Part model, mm, in its own coordinate system. Face numbers are marked on the shaded views. A direction names the side the tool comes from. Round coordinates to 2 decimals unless told otherwise and drop trailing zeros. Write each loop counter-clockwise with the first axis right and the second up, starting at its lowest first coordinate (ties: lowest second). Pieces come first, ordered by that corner, then holes.
```python
from build123d import *

# Parameters (mm, degrees)
FILLET2_R = 50.8
FILLET3_R = 7.62


with BuildPart() as part:
    # Sketch1 → Revolve1 (revolve)
    with BuildSketch(Plane(origin=(0, 0, 0), x_dir=(1, 0, 0), z_dir=(0, 1, 0)), mode=Mode.PRIVATE) as revolve1_sk:
        Polygon((-78.74, 0), (-61.722, 0), (-61.722, 147.1422), (0, 147.1422), (0, 294.2844), (-62.23, 294.2844), (-62.23, 249.0724), (-129.54, 249.0724), (-129.54, 37.846), (-78.74, 37.846), align=None)
    revolve(revolve1_sk.sketch.rotate(Axis((0, 0, 0), (0, 0, -1)), 180), axis=Axis((0, 0, 0), (0, 0, -1)))

    # Fillet2
    fillet2_edges = [part.edges().sort_by_distance(p)[0] for p in [
        (-129.54, 0, -37.846),
        (-129.54, 0, -249.0724),
    ]]
    fillet(fillet2_edges, radius=FILLET2_R - 0.0001)  # a hair under: the kernel refuses the full size

    # Fillet3
    fillet3_edges = [part.edges().sort_by_distance(p)[0] for p in [
        (-62.23, 0, -294.2844),
    ]]
    fillet(fillet3_edges, radius=FILLET3_R)


solid = part.part
```
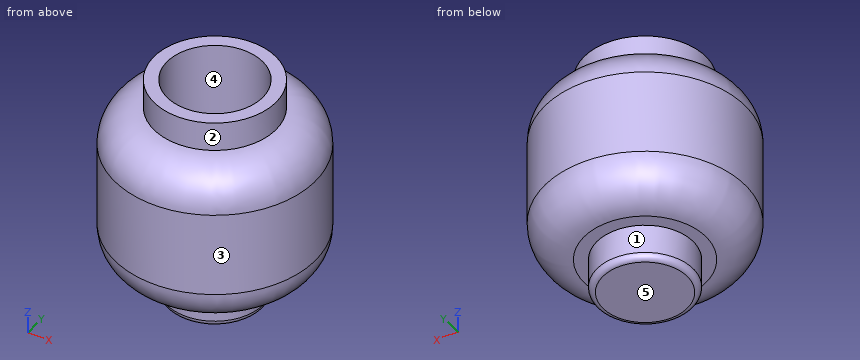
Q1. Cut at D-D on z = -269.5. Write the cut outline in (x, y).
Values follow:
outline: circle Ø124.46 at (0, 0)
Q2. Mould opens along X. For the marked faces 3, 4 and 5 say: +X half, -X half, draft (parallel to the pull), parting line (faces both ways), or undercut.
Values follow:
face 3: parting line
face 4: undercut
face 5: draft
Q3. Wall check: L1, parallel to Y at x = -50, z = -26; L2, parallel to Y at x = 42, z = -78; L3, parallel to Z at x = 3, y = 2.5. Give the ranges that are in metal, low to high.
Values follow:
L1: y = -60.83 to -36.19, 36.19 to 60.83
L2: y = -121.35 to -45.23, 45.23 to 121.35
L3: z = -294.28 to -147.14
Q4. Which spindle directions (+Z, -Z, +X, -X, +Y, -Y) get a long thin tool onto all of the face, cutting with end or side? Do the marked faces 1 and 2. Say none if no direction does.
Values follow:
face 1: -Z
face 2: +Z
Q5. Cut at C-C on z = -177.5. Write the cut outline in (x, y), plus the area to 3 significant figures.
Values follow:
outline: circle Ø259.08 at (0, 0)
area: 52,700 mm2
Q6. Drop flat-ended pins along their axis: pin 1 (8 mm diameter, centred on x = -27.5, z = -187, fed in from -Y); pin 2 (10 mm diameter, centred on x = -36, z = -57.5, fed in from +Y); pin 3 (2 mm diameter, centred on x = -78, y = 98, fed in from -Z). Give the stop position or say it passes through.
Values follow:
pin 1: stops at y = -127.39
pin 2: stops at y = 117.21
pin 3: stops at z = -220.84
